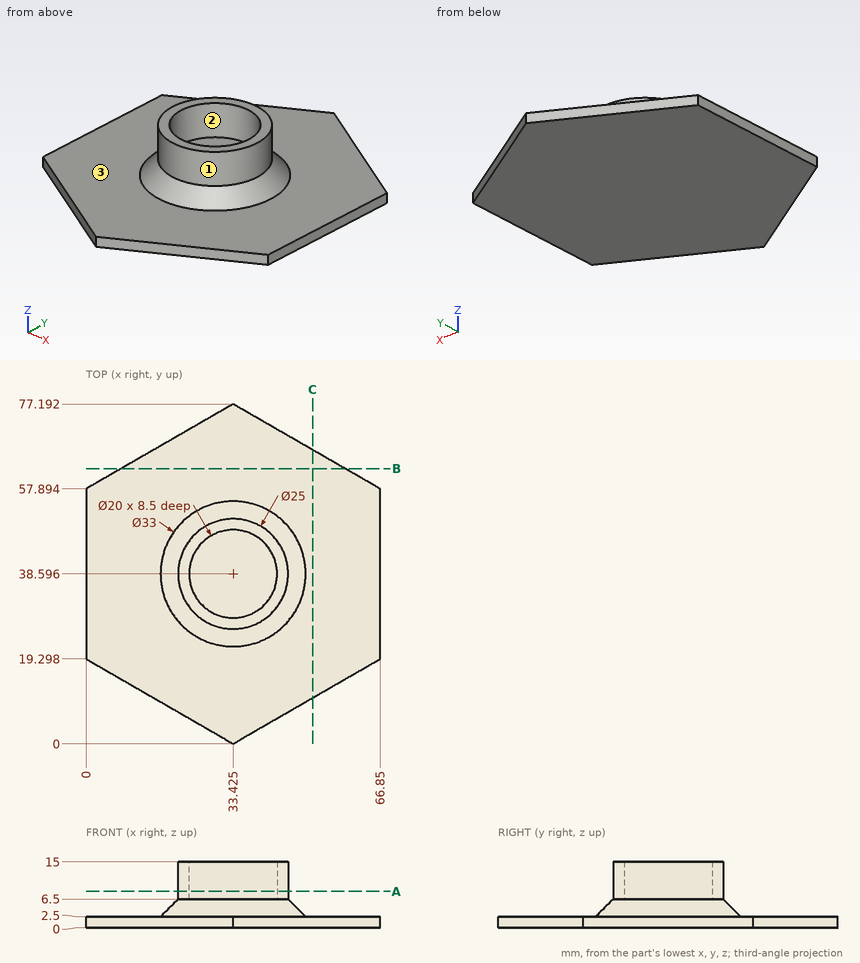
Design review of the part shown in the three views and the two pictorial views. Dimensions are in mm from the part's minimum x, y and z. Coordinates: 2 decimals unless noted, no trailing zeros. Order: outer loops, then holes, each group sorted by start corner. A loop starts at its lowest first (then second) coordinate and runs counter-clockwise, first axis right, second up.
1) Take a section at B-B, the plane y = 62.5. Give the boundary of the cut face in (x, z).
2) Take a section at A-A, the plane z = 8.25. Give the boundary of the cut face in (x, y) (1 decimal).
3) Take a section at C-C, the plane x = 51.5. Give the boundary of the cut face in (y, z), and give its area (3 significant figures).
4) Mouldability with a two-part tool opening along X and no side actions: class the marked faces 1, 2 and 3 as +X half, -X half, draft (parallel to the pull), parting line (faces both ways), or undercut.
5) Clearance check with flat-ended pins moving along their axes: pin 1 (12 mm diameter, centred on x = 26.5, y = 11.5, fed in from +Z); pin 2 (1 mm diameter, centred on x = 45, z = 10, fed in from -Y); pin 3 (4 mm diameter, centred on x = 24.5, z = 4, fed in from +Y). State where each tip first meets the part, or that it passes through.
6) Wall thickness on line 1 along X through (y, z) = (38.5, 8.25) (1 decimal); line 2 along Y through (x, z) = (29, 12.25) (1 decimal); line 3 along Y through (x, z) = (26.5, 9.5): over which ranges is each line inside the solid? List them lowest first.
Returned:
1. outline: (7.98, 0) - (58.87, 0) - (58.87, 2.5) - (7.98, 2.5) - close
2. outline: circle Ø25 at (33.4, 38.6); hole circle Ø20 at (33.4, 38.6)
3. outline: (10.44, 0) - (66.76, 0) - (66.76, 2.5) - (10.44, 2.5) - close
3. area: 141 mm2
4. face 1: parting line
4. face 2: undercut
4. face 3: draft
5. pin 1: stops at z = 2.5
5. pin 2: stops at y = 32.8
5. pin 3: stops at y = 72.8
6. line 1: x = 20.9 to 23.4, 43.4 to 45.9
6. line 2: y = 26.9 to 29.6, 47.6 to 50.3
6. line 3: y = 28.19 to 31.38, 45.81 to 49
